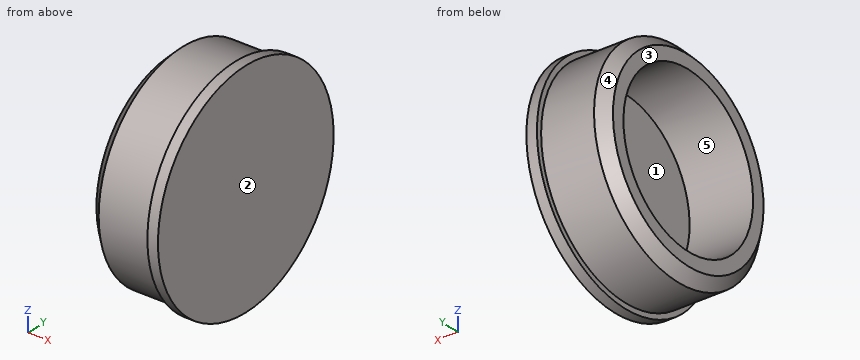
```python
from build123d import *

# Parameters (mm, degrees)
ESQUISSE1_R      = 10.5
EXTRUSION1_DEPTH = 1
ESQUISSE2_R      = 10
ESQUISSE2_R_2    = 7.75
EXTRUSION2_DEPTH = 6
CHANFREIN1_SIZE  = 1


with BuildPart() as part:
    # Esquisse1 → Extrusion1 (new body)
    with BuildSketch(Plane(origin=(0, 0, 0), x_dir=(0, 0, -1), z_dir=(1, 0, 0))):
        Circle(ESQUISSE1_R)
    extrude(amount=EXTRUSION1_DEPTH)

    # Esquisse2 → Extrusion2 (add)
    with BuildSketch(Plane.ZY):
        with Locations(Location((0, 0, 0), (0, 0, 180))):  # turned: the seam where the file's is
            Circle(ESQUISSE2_R)
        Circle(ESQUISSE2_R_2, mode=Mode.SUBTRACT)
    extrude(amount=EXTRUSION2_DEPTH)

    # Chanfrein1
    chanfrein1_edges = [part.edges().sort_by_distance(p)[0] for p in [
        (-6, 0, 10),
    ]]
    chamfer(chanfrein1_edges, length=CHANFREIN1_SIZE)


solid = part.part
```
Source: CAD feature listing. Evaluate the final solid. Frame: model axes, mm. Face numbers are marked on the shaded views. A direction names the side the tool comes from. Coordinates: 2 decimals unless noted, no trailing zeros. Write each loop counter-clockwise with the first axis right and the second up, starting at its lowest first coordinate (ties: lowest second). Pieces come first, ordered by that corner, then holes. Notation, with made-up numbers: (-33.75, -0.75) - (6.25, -0.75) arc R23 ccw to (6.25, 22.25) - close; hole circle Ø4 at (12, 48). An arc over 180 degrees is marked (long way). Answer as a JSON object with one key per item and string values.
Q1. First-contact query: pin 1 Ø1.5 at (x, y) = (-1.5, -8) entering from +Z; pin 2 Ø10.5 at (y, z) = (0.5, 0) entering from -X; pin 3 Ø2 at (x, y) = (-2.5, 7.5) entering from -Z. Flat tips, straight axial feed; report the tip coordinate or a pass-through.
Ans:
{"pin 1": "stops at z = 6.89", "pin 2": "stops at x = 0", "pin 3": "stops at z = -7.6"}
Q2. Material intervals for line 1 (Y direction, x = -3.9, z = 0); line 2 (X direction, y = 5.25, z = 4.75); line 3 (Z direction, x = -1.5, y = -4.75), sorted ascending. Write a range as [from, to].
Ans:
{"line 1": "y = [-10, -7.75], [7.75, 10]", "line 2": "x = [0, 1]", "line 3": "z = [-8.8, -6.12], [6.12, 8.8]"}
Q3. Set-up query: the marked faces 1 and 2. Return all of +Z, -Z, +X, -X, +Y, -Y with unobstructed straight access to the full face (end or side cutting, diameter ignored); none if empty.
Ans:
{"face 1": "-X", "face 2": "+Z, -Z, +X, +Y, -Y"}
Q4. Section query A-A, the plane y = 0. Output: boundary loops of the cut face in (x, z), plus the area to 3 significant figures.
Ans:
{"outline": "(-6, -9) - (-5, -10) - (0, -10) - (0, -10.5) - (1, -10.5) - (1, 10.5) - (0, 10.5) - (0, 10) - (-5, 10) - (-6, 9) - (-6, 7.75) - (0, 7.75) - (0, -7.75) - (-6, -7.75) - close", "area": "47.0 mm2"}
Q5. Section query C-C, the plane x = -4. Output: boundary loops of the cut face in (y, z).
Ans:
{"outline": "circle Ø20 at (0, 0); hole circle Ø15.5 at (0, 0)"}
Q6. Draft query along Z for the marked faces 3, 4 and 5. Return one class per face: released by +Z, released by -Z, zero draft, split by the parting line, or undercut.
Ans:
{"face 3": "zero draft", "face 4": "split by the parting line", "face 5": "undercut"}
